Read the model definition and answer for the solid it produces. Units are mm, in the model's axes. A direction names the side the tool comes from. Round coordinates to 2 decimals unless told otherwise and drop trailing zeros. Order: outer loops, then holes, each group sorted by start corner. A loop starts at its lowest first (then second) coordinate and runs counter-clockwise, first axis right, second up. Notation, with made-up numbers: (50, -17) - (78, -17) arc R18 cw to (78, 0) - close; hole circle Ø3 at (65.5, 58). An arc over 180 degrees is marked (long way). Answer as a JSON object with one key per item and string values. Group by question number.
Q1. A cutting plane is placed at D-D on y = -1.7. Determine the outline of the cut face in (x, z) (3 decimals).
Q2. Consider line 1 (Z direction, x = 9.75, y = 1.8); line 2 (Z direction, x = 9.25, y = 0.65); line 3 (Y direction, x = -1.75, z = -8). Determine where each line is inside the solid, lowest interval first.
Q3. A cutting plane is placed at C-C on x = -7.62. Determine the outline of the cut face in (y, z).
Q4. A tool of negligible diameter and unlimited length cuts with its end or side. For faces 4 (the cylindrical face through (6.967, 1.002, 0.34)), 5 (the flat face through (3, 2.032, -3)), from which of +Z, -Z, +X, -X, +Y, -Y can it reach the whole face along a straight path? Write none if from no direction.
Q5. Given pin 1 Ø1.7 at (x, z) = (-9.47, -3.3) entering from -Y; pin 2 Ø2.5 at (x, z) = (-7.24, -2.39) entering from +Y; pin 3 Ø3 at (x, z) = (0, 0) entering from +Y; pin 4 Ø1.2 at (x, z) = (0, -8.509) entering from +Y, each flat-ended and moving along its own axis, determine where each tip first touches the part or whether it passes through.
Q6. The mould has two halves that part along X. Classify faces 1 (the cylindrical face through (10.763, 1.002, -0.096)), 2 (the flat face through (-1, 2.464, -3)), 3 (the cylindrical face through (0.96, -1.24, 4.34)): pulls with the +X half, pulls with the -X half, needs draft (parallel to the pull), parting line crosses it, or undercut.
Q7. A cutting plane is placed at A-A on z = 0. Count the separate pieces of the cut face and the enclosed holes in it, and give its area (3 significant figures).
```python
from build123d import *

# Parameters (mm, degrees)
SKETCH1_R           = 12.0015
SKETCH1_R_2         = 0.7366
SKETCH1_R_3         = 3.81
BOSS_EXTRUDE1_DEPTH = 2.032


with BuildPart() as part:
    # Sketch1 → Boss-Extrude1 (new body)
    with BuildSketch(Plane(origin=(0, 0, 0), x_dir=(1, 0, 0), z_dir=(0, 1, 0))):
        with Locations(Location((0, 0, 0), (0, 0, 270))):
            Circle(SKETCH1_R)
        with Locations(Location((0, 8.509, 0), (0, 0, 90))):
            Circle(SKETCH1_R_2, mode=Mode.SUBTRACT)
        with Locations(Location((0, -8.509, 0), (0, 0, 90))):
            Circle(SKETCH1_R_2, mode=Mode.SUBTRACT)
        with Locations(Location((7.62, 0, 0), (0, 0, 270))):
            Circle(SKETCH1_R_2, mode=Mode.SUBTRACT)
        with Locations(Location((-7.62, 0, 0), (0, 0, 90))):
            Circle(SKETCH1_R_2, mode=Mode.SUBTRACT)
        with Locations(Location((2.8575, -8.014847145, 0), (0, 0, 270))):
            Circle(SKETCH1_R_2, mode=Mode.SUBTRACT)
        with Locations(Location((2.8575, 8.014847145, 0), (0, 0, 270))):
            Circle(SKETCH1_R_2, mode=Mode.SUBTRACT)
        with Locations(Location((-2.8575, -8.014847145, 0), (0, 0, 90))):
            Circle(SKETCH1_R_2, mode=Mode.SUBTRACT)
        with Locations(Location((-2.8575, 8.014847145, 0), (0, 0, 90))):
            Circle(SKETCH1_R_2, mode=Mode.SUBTRACT)
        with Locations(Location((7.236281244, 2.3876, 0), (0, 0, 270))):
            Circle(SKETCH1_R_2, mode=Mode.SUBTRACT)
        with Locations(Location((7.236281244, -2.3876, 0), (0, 0, 270))):
            Circle(SKETCH1_R_2, mode=Mode.SUBTRACT)
        with Locations(Location((9.474063806, 3.302, 0), (0, 0, 270))):
            Circle(SKETCH1_R_2, mode=Mode.SUBTRACT)
        with Locations(Location((9.474063806, -3.302, 0), (0, 0, 270))):
            Circle(SKETCH1_R_2, mode=Mode.SUBTRACT)
        with Locations(Location((-7.236281244, -2.3876, 0), (0, 0, 90))):
            Circle(SKETCH1_R_2, mode=Mode.SUBTRACT)
        with Locations(Location((-9.474063806, -3.302, 0), (0, 0, 90))):
            Circle(SKETCH1_R_2, mode=Mode.SUBTRACT)
        with Locations(Location((-9.474063806, 3.302, 0), (0, 0, 90))):
            Circle(SKETCH1_R_2, mode=Mode.SUBTRACT)
        with Locations(Location((-7.236281244, 2.3876, 0), (0, 0, 90))):
            Circle(SKETCH1_R_2, mode=Mode.SUBTRACT)
        with Locations(Location((10.033, 0, 0), (0, 0, 270))):
            Circle(SKETCH1_R_2, mode=Mode.SUBTRACT)
        with Locations(Location((-10.033, 0, 0), (0, 0, 270))):
            Circle(SKETCH1_R_2, mode=Mode.SUBTRACT)
        with Locations(Location((0, 0, 0), (0, 0, 270))):
            Circle(SKETCH1_R_3, mode=Mode.SUBTRACT)
    extrude(amount=BOSS_EXTRUDE1_DEPTH)

    # Sketch3 → hub (revolve)
    with BuildSketch(Plane.XY, mode=Mode.PRIVATE) as hub_sk:
        Polygon((1.3843, 0.5334), (2.794, 0.5334), (2.794, -2.5146), (4.445, -2.5146), (4.445, 0), (3.7465, 0), (3.7465, 2.4638), (2.9972, 2.4638), (2.9972, 1.2446), (1.3843, 1.2446), align=None)
    revolve(hub_sk.sketch.rotate(Axis((0, 2.4638, 0), (0, -1, 0)), 180), axis=Axis((0, 2.4638, 0), (0, -1, 0)))


solid = part.part
```
Result set:
{
 "1": {"outline": "circle Ø8.89 at (0, 0); hole circle Ø5.588 at (0, 0)"},
 "2": {"line 1": "z = -7 to -3.98, -2.62 to -0.68, 0.68 to 2.62, 3.98 to 7", "line 2": "z = -7.65 to -4, -2.6 to 2.6, 4 to 7.65", "line 3": "y = 0 to 2.03"},
 "3": {"outline": "(0, -9.27) - (2.03, -9.27) - (2.03, -3.02) - (0, -3.02) - close; (0, -1.76) - (2.03, -1.76) - (2.03, -0.74) - (0, -0.74) - close; (0, 0.74) - (2.03, 0.74) - (2.03, 1.76) - (0, 1.76) - close; (0, 3.02) - (2.03, 3.02) - (2.03, 9.27) - (0, 9.27) - close"},
 "4": {"face 4": "+Y, -Y", "face 5": "+Y"},
 "5": {"pin 1": "stops at y = 0", "pin 2": "stops at y = 2.03", "pin 3": "stops at y = 1.24", "pin 4": "passes through"},
 "6": {"face 1": "undercut", "face 2": "needs draft", "face 3": "parting line crosses it"},
 "7": {"separate pieces": "6", "enclosed holes": "0", "area": "35.8 mm²"}
}
